from build123d import *


with BuildPart() as part:
    # Sketch1 → Revolve1 (revolve)
    with BuildSketch(Plane.XY, mode=Mode.PRIVATE) as revolve1_sk:
        with BuildLine():
            Line((-14.5, 0), (14.5, 0))
            Line((14.5, 0), (14.5, 3))
            Line((14.5, 3), (27.5, 3))
            Line((27.5, 3), (27.5, 7.5))
            Line((27.5, 7.5), (9.972135955, 7.5))
            ThreePointArc((9.972135955, 7.5), (9.512630114, 7.446497979), (9.077708764, 7.288854382))
            Line((9.077708764, 7.288854382), (6.922291236, 6.211145618))
            ThreePointArc((6.922291236, 6.211145618), (6.487369886, 6.053502021), (6.027864045, 6))
            Line((6.027864045, 6), (-6.027864045, 6))
            ThreePointArc((-6.027864045, 6), (-6.487369886, 6.053502021), (-6.922291236, 6.211145618))
            Line((-6.922291236, 6.211145618), (-9.077708764, 7.288854382))
            ThreePointArc((-9.077708764, 7.288854382), (-9.512630114, 7.446497979), (-9.972135955, 7.5))
            Line((-9.972135955, 7.5), (-27.5, 7.5))
            Line((-27.5, 7.5), (-27.5, 3))
            Line((-27.5, 3), (-14.5, 3))
            Line((-14.5, 3), (-14.5, 0))
        make_face()
    revolve(revolve1_sk.sketch.rotate(Axis((-44.087306847, 0, 0), (1, 0, 0)), 90), axis=Axis((-44.087306847, 0, 0), (1, 0, 0)))


solid = part.part
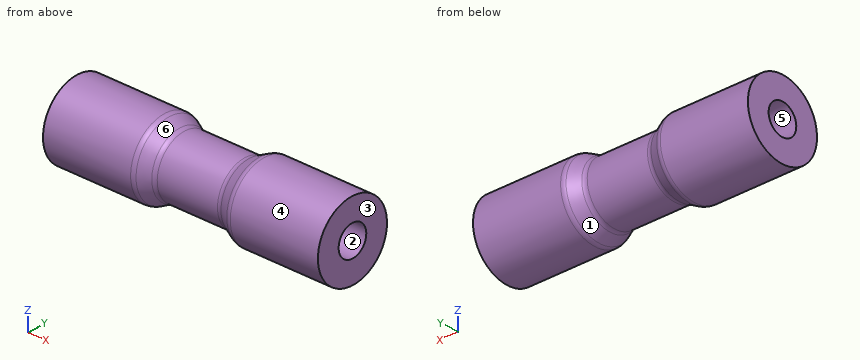
Could you check a few things on this model? Use its own coordinates, in mm. Face numbers are marked on the shaded views. A direction names the side the tool comes from. Coordinates: 2 decimals unless noted, no trailing zeros. Order: outer loops, then holes, each group sorted by start corner. A loop starts at its lowest first (then second) coordinate and runs counter-clockwise, first axis right, second up.
Q1. Suppose I cut it at C-C on x = 17. Please give me the cut outline in (y, z).
Q2. Which directions (+Z, -Z, +X, -X, +Y, -Y) give clear straight access to the entire face, cutting with the end or side of a thin tool? Please do the marked faces 4, 5 and 6.
Q3. Will these pins go through, and if not, where does the flat tip stop? pin 1 (6.5 mm diameter, centred on y = 1, z = -0.5, fed in from +X); pin 2 (5 mm diameter, centred on x = -3, y = -4, fed in from +Z); pin 3 (5.5 mm diameter, centred on y = 0, z = 0, fed in from +X); pin 4 (5 mm diameter, centred on x = -19, z = -3.5, fed in from -Y).
Q4. Thinking about a two-plate mould opening in X: for the marked faces 1, 2 and 3, which applies, released by +X, released by -X, zero draft, split by the parting line, or undercut?
Q5. Suppose I cut it at D-D on x = -13.5. Please give me the cut outline in (y, z), and give its area (3 significant figures).
Q6. Suppose I cut it at A-A on y = 0. Please give me the cut outline in (x, z), and give its area (3 significant figures).
Q7. Please list where these lines run through material, in increasing order: L1, parallel to Y at x = -22.5, z = 0; L2, parallel to Y at x = -17, z = 4.5; L3, parallel to X at y = -4.25, z = 5.75.
Answer:
1. outline: circle Ø15 at (0, 0); hole circle Ø6 at (0, 0)
2. face 4: +X, -X
2. face 5: -X
2. face 6: none
3. pin 1: stops at x = 27.5
3. pin 2: stops at z = 5.81
3. pin 3: stops at x = 14.5
3. pin 4: stops at y = -7.43
4. face 1: undercut
4. face 2: zero draft
4. face 3: released by +X
5. outline: circle Ø15 at (0, 0)
5. area: 177 mm2
6. outline: (-27.5, -7.5) - (-9.97, -7.5) arc R2 ccw to (-9.08, -7.29) - (-6.92, -6.21) arc R2 cw to (-6.03, -6) - (6.03, -6) arc R2 cw to (6.92, -6.21) - (9.08, -7.29) arc R2 ccw to (9.97, -7.5) - (27.5, -7.5) - (27.5, -3) - (14.5, -3) - (14.5, 3) - (27.5, 3) - (27.5, 7.5) - (9.97, 7.5) arc R2 ccw to (9.08, 7.29) - (6.92, 6.21) arc R2 cw to (6.03, 6) - (-6.03, 6) arc R2 cw to (-6.92, 6.21) - (-9.08, 7.29) arc R2 ccw to (-9.97, 7.5) - (-27.5, 7.5) - (-27.5, 3) - (-14.5, 3) - (-14.5, -3) - (-27.5, -3) - close
6. area: 621 mm2
7. L1: y = -7.5 to -3, 3 to 7.5
7. L2: y = -6 to 6
7. L3: x = -27.5 to -8.8, 8.8 to 27.5
